from build123d import *

# Parameters (mm, degrees)
EXTRUDE_THIN1_DEPTH   = 3
SKETCH1_3_R           = 3
BOSS_EXTRUDE1_DEPTH   = 3
FILLET1_R             = 5
F_2_5MM_DOWEL_HOLE1_D = 2.5
CHAMFER1_SIZE         = 0.25


with BuildPart() as part:
    # Sketch1 → Extrude-Thin1 (new body)
    with BuildSketch(Plane.XY):
        with BuildLine():
            ThreePointArc((67.801370449, 34.141342947), (56.598136233, 33.812681852), (47.198138914, 27.708541828))
            ThreePointArc((47.198138914, 27.708541828), (40.574587763, 23.069242721), (32.560988498, 21.984460302))
            Line((32.560988498, 21.984460302), (18.0194176, 23.497567077))
            ThreePointArc((18.0194176, 23.497567077), (10.297542455, 21.776854665), (5.1667157, 15.754992513))
            Line((5.1667157, 15.754992513), (-0.737799909, 1.088733357))
            Line((-0.737799909, 1.088733357), (2.04513605, -0.031653828))
            Line((2.04513605, -0.031653828), (7.949651659, 14.634605328))
            ThreePointArc((7.949651659, 14.634605328), (11.845577871, 19.207110251), (17.7089323, 20.513677186))
            Line((17.7089323, 20.513677186), (32.250503198, 19.000570412))
            ThreePointArc((32.250503198, 19.000570412), (41.667206568, 20.275287791), (49.450477778, 25.726883522))
            ThreePointArc((49.450477778, 25.726883522), (57.492238313, 30.949016112), (67.076680067, 31.230187876))
            Line((67.076680067, 31.230187876), (67.801370449, 34.141342947))
        make_face()
    extrude(amount=EXTRUDE_THIN1_DEPTH)

    # Sketch1<3> → Boss-Extrude1 (add, through all)
    with BuildSketch(Plane.XY):
        with Locations((0.653668071, 0.528539764)):
            Circle(SKETCH1_3_R)
        with Locations((67.439025258, 32.685765412)):
            Circle(SKETCH1_3_R)
    extrude(amount=BOSS_EXTRUDE1_DEPTH)

    # Fillet1
    fillet1_edges = [part.edges().sort_by_distance(p)[0] for p in [
        (0.232483855, 3.498826595, 1.5),
        (3.015419815, 2.37843941, 1.5),
        (64.619351463, 31.661343773, 1.5),
        (65.147115394, 34.621520866, 1.5),
    ]]
    fillet(fillet1_edges, radius=FILLET1_R)

    # Ø2.5mm Dowel Hole1 (through all)
    with Locations(Plane.XY.offset(3)):
        with Locations((67.439025258, 32.685765412), (0.653668071, 0.528539764)):
            Hole(F_2_5MM_DOWEL_HOLE1_D / 2)

    # Chamfer1
    chamfer1_edges = [part.edges().sort_by_distance(p)[0] for p in [
        (10.297542455, 21.776854665, 0),
        (25.290203049, 22.741013689, 0),
        (40.574587763, 23.069242721, 0),
        (41.667206568, 20.275287791, 0),
        (24.979717749, 19.757123799, 0),
        (5.868250185, 9.464600631, 3),
        (11.845577871, 19.207110251, 0),
        (5.868250185, 9.464600631, 0),
        (3.085314225, 10.584987816, 0),
        (11.845577871, 19.207110251, 3),
        (24.979717749, 19.757123799, 3),
        (41.667206568, 20.275287791, 3),
        (40.574587763, 23.069242721, 3),
        (25.290203049, 22.741013689, 3),
        (10.297542455, 21.776854665, 3),
        (3.085314225, 10.584987816, 3),
        (55.029480027, 29.973141473, 0),
        (55.029480027, 29.973141473, 3),
        (70.417176443, 32.324357726, 0),
        (70.417176443, 32.324357726, 3),
        (54.557553661, 33.056070888, 0),
        (54.557553661, 33.056070888, 3),
        (-0.466719115, -2.254396195, 3),
        (-0.466719115, -2.254396195, 0),
        (63.752058153, 31.452795933, 3),
        (63.752058153, 31.452795933, 0),
        (64.7995305, 34.870879047, 3),
        (64.7995305, 34.870879047, 0),
        (3.437869945, 2.784750939, 0),
        (3.437869945, 2.784750939, 3),
        (0.209401135, 4.084505995, 0),
        (0.209401135, 4.084505995, 3),
    ]]
    chamfer(chamfer1_edges, length=CHAMFER1_SIZE - 0.0001)  # a hair under: the kernel refuses the full size


solid = part.part
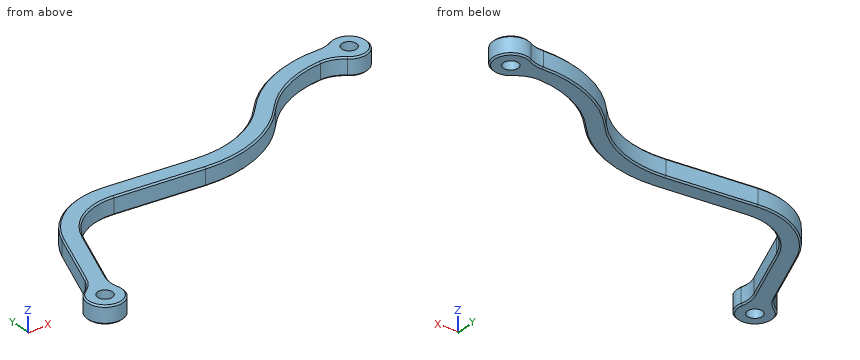
Could you check a few things on this model? Use its own coordinates, in mm. Give positions to 0.01 mm unless a question says otherwise; leave off trailing zeros. Write each loop counter-clockwise with the first axis right and the second up, starting at its lowest first coordinate (ties: lowest second). Pieces come first, ordered by that corner, then holes. Notation, with made-up numbers: (38, 63.25) - (67, 63.25) arc R24 ccw to (67, 82.25) - close; hole circle Ø7 at (5, 5.5). An arc over 180 degrees is marked (long way). Use CSV: the item, a comma, the result in double quotes. Start each with the question number.
Item 1: If I drill on line 1 along X through (y, z) = (0.5, 0.3); line 2 along Y through (x, z) = (35, 1); line 3 along Y through (x, z) = (16.5, 0.45), over which ranges is the centre line in solid material (lowest first)?
Item 2: I want a section at A-A, the plane y = 8. Please give me the cut outline in (x, z), then the cut area to 3 significant figures.
Item 3: I'm going to push flat-ended pins straight in: pin 1 (1.5 mm diameter, centred on x = 50.5, z = 1.5, fed in from -Y); pin 2 (3 mm diameter, centred on x = 67.44, y = 32.69, fed in from +Z); pin 3 (1.5 mm diameter, centred on x = 42.5, z = 2.5, fed in from -Y). Where does each tip first touch, or does it pass through?
Item 4: I want a section at B-B, the plane z = 1.75. Give the number of separate pieces and of enclosed holes in the cut face, then the cut area to 3 significant figures.
Findings:
1,line 1,"x = -2.35 to -0.6, 1.9 to 3.65"
1,line 2,"y = 18.9 to 21.91"
1,line 3,"y = 20.56 to 23.56"
2,outline,"(2.04, 0.25) - (2.31, 0) - (5.01, 0) - (5.28, 0.25) - (5.28, 2.75) - (5.01, 3) - (2.31, 3) - (2.04, 2.75) - close"
2,area,"9.57 mm2"
3,pin 1,"stops at y = 26.06"
3,pin 2,"stops at z = 3"
3,pin 3,"stops at y = 20.31"
4,separate pieces,"1"
4,enclosed holes,"2"
4,area,"282 mm2"
